Check sheet for the modelled part. Datum: model origin and axes. Units: mm. Face numbers are marked on the shaded views. A direction names the side the tool comes from. Give positions to 0.01 mm unless a question says otherwise; leave off trailing zeros. Loops run counter-clockwise (first coordinate to the right, second up) from the corner with the lowest first, then second, coordinate; pieces in that order, holes last. Notation, with made-up numbers: M 65.25,63 L 77.25,63 A27 cw 77.25,101 Z; hole C -17.75,-10.75 d9. An arc over 180 degrees is marked long. One line per question, with ' | ' between items. Start each with the question number.
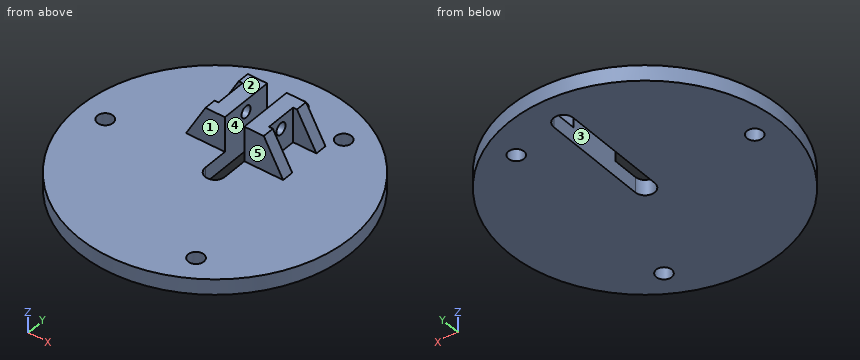
from build123d import *

# Parameters (mm, degrees)
SKETCH_1_R          = 35
SKETCH_1_R_2        = 2
EXTRUDE_1_DEPTH     = 4
EXTRUDE_2_DEPTH     = 9
CUT_EXTRUDE_1_DEPTH = 14
SKETCH_4_R          = 1.45
CUT_EXTRUDE_2_DEPTH = 13
SKETCH_5_R          = 1.5
CUT_EXTRUDE_3_DEPTH = 13


with BuildPart() as part:
    # 草图1 → 凸台-拉伸1 (new body)
    with BuildSketch(Plane.XY):
        Circle(SKETCH_1_R)
        with Locations((14.125, 24.465217657)):
            Circle(SKETCH_1_R_2, mode=Mode.SUBTRACT)
        with Locations((14.125, -24.465217657)):
            Circle(SKETCH_1_R_2, mode=Mode.SUBTRACT)
        with Locations((-28.25, 0)):
            Circle(SKETCH_1_R_2, mode=Mode.SUBTRACT)
        with BuildLine():
            Line((-2.5, 0), (-2.5, 27))
            ThreePointArc((-2.5, 27), (0, 29.5), (2.5, 27))
            Line((2.5, 27), (2.5, 0))
            ThreePointArc((2.5, 0), (0, -2.5), (-2.5, 0))
        make_face(mode=Mode.SUBTRACT)
    extrude(amount=EXTRUDE_1_DEPTH)

    # 草图2 → 凸台-拉伸2 (add)
    with BuildSketch(Plane.XY.offset(4)):
        Polygon((-2.5, 13.5), (-2.5, 20.5), (-12.5, 20.5), (-12.5, 17.5), (-6.5, 17.5), (-6.5, 9.5), (-12.5, 9.5), (-12.5, 6.5), (-2.5, 6.5), align=None)
        Polygon((2.5, 6.5), (2.5, 13.5), (2.5, 20.5), (12.5, 20.5), (12.5, 17.5), (6.5, 17.5), (6.5, 9.5), (12.5, 9.5), (12.5, 6.5), align=None)
    extrude(amount=EXTRUDE_2_DEPTH)

    # 草图3 → 切除-拉伸1 (cut)
    with BuildSketch(Plane.XZ.offset(-6.5)):
        Polygon((-12.5, 4), (-12.5, 13), (-7.5, 13), align=None)
        Polygon((12.5, 4), (12.5, 13), (7.5, 13), align=None)
    extrude(amount=-CUT_EXTRUDE_1_DEPTH, mode=Mode.SUBTRACT)

    # 草图4 → 切除-拉伸2 (cut)
    with BuildSketch(Plane.ZY.offset(6.5)):
        with Locations((10, 13.5)):
            Circle(SKETCH_4_R)
    extrude(amount=-CUT_EXTRUDE_2_DEPTH, mode=Mode.SUBTRACT)

    # 草图5 → 切除-拉伸3 (cut)
    with BuildSketch(Plane(origin=(6.5, 0, 0), x_dir=(0, 0, -1), z_dir=(1, 0, 0))):
        with Locations((-10, 13.5)):
            Circle(SKETCH_5_R)
    extrude(amount=-CUT_EXTRUDE_3_DEPTH, mode=Mode.SUBTRACT)


solid = part.part
Q1. Depth check by flat-ended pin: P1, Ø4, axis at x = -19, y = 9, coming from the +Z side; P2, Ø5, axis at x = 1.5, y = 20, coming from the -Z side; P3, Ø4, axis at y = 13.5, z = 7.5, coming from the -X side; P4, Ø4.5, axis at x = -9, z = 10.5, coming from the -Y side. Enter the tip coordinate at first touch or a pass-through.
Q2. Cross-section at A-A (x = 0). Record the cut outline in (y, z).
Q3. Draft check along X on the marked faces 3, 4 and 5. Enter one of: released by +X, released by -X, zero draft, split by the parting line, or undercut.
Q4. Access from +Z, -Z, +X, -X, +Y, -Y to the whole of each face (thin tool, end or side, straight path). Record for the marked faces 1 and 2.
Q5. Cross-section at C-C (z = 6.5). Record the cut outline in (x, y), and give its area (3 significant figures).
Q6. Material ranges on probe 1 along Y at (x, z) = (-3.5, 10); probe 2 along Z at (x, y) = (-30, -10); probe 3 along X at (y, z) = (11.5, 2.75), recorded low to high. Write a range as from..to.
Q7. Cross-section at B-B (y = 13.5). Record the cut outline in (x, z), and give its area (3 significant figures).
Q8. Cross-section at D-D (z = 10). Record the cut outline in (x, y), and give its area (3 significant figures).
Solved:
1) P1: stops at z = 4 | P2: stops at z = 0 | P3: stops at x = -6.5 | P4: stops at y = 6.5
2) outline: M -35,0 L -2.5,0 L -2.5,4 L -35,4 Z; M 29.5,0 L 35,0 L 35,4 L 29.5,4 Z
3) face 3: undercut | face 4: undercut | face 5: zero draft
4) face 1: +Z, +X, -X, -Y | face 2: +Z, +X, -X, +Y, -Y
5) outline: M -11.11,6.5 L -2.5,6.5 L -2.5,20.5 L -11.11,20.5 L -11.11,17.5 L -6.5,17.5 L -6.5,9.5 L -11.11,9.5 Z; M 2.5,6.5 L 11.11,6.5 L 11.11,9.5 L 6.5,9.5 L 6.5,17.5 L 11.11,17.5 L 11.11,20.5 L 2.5,20.5 Z | area: 167 mm²
6) probe 1: y = 6.5..12, 15..20.5 | probe 2: z = 0..4 | probe 3: x = -33.06..-2.5, 2.5..33.06
7) outline: M -32.29,0 L -2.5,0 L -2.5,8.5 L -6.5,8.5 L -6.5,4 L -32.29,4 Z; M -6.5,11.5 L -2.5,11.5 L -2.5,13 L -6.5,13 Z; M 2.5,0 L 32.29,0 L 32.29,4 L 6.5,4 L 6.5,8.5 L 2.5,8.5 Z; M 2.5,11.5 L 6.5,11.5 L 6.5,13 L 2.5,13 Z | area: 286 mm²
8) outline: M -9.17,6.5 L -2.5,6.5 L -2.5,12 L -6.5,12 L -6.5,9.5 L -9.17,9.5 Z; M -9.17,17.5 L -6.5,17.5 L -6.5,15 L -2.5,15 L -2.5,20.5 L -9.17,20.5 Z; M 2.5,6.5 L 9.17,6.5 L 9.17,9.5 L 6.5,9.5 L 6.5,12 L 2.5,12 Z; M 2.5,15 L 6.5,15 L 6.5,17.5 L 9.17,17.5 L 9.17,20.5 L 2.5,20.5 Z | area: 120 mm²
